from build123d import *

# Parameters (mm, degrees)
SKETCH1_W           = 5
SKETCH1_H           = 13
BOSS_EXTRUDE1_DEPTH = 2.5
SKETCH2_R           = 3
BOSS_EXTRUDE2_DEPTH = 5


with BuildPart() as part:
    # Sketch1 → Boss-Extrude1 (new body)
    with BuildSketch(Plane(origin=(0, 0, 0), x_dir=(1, 0, 0), z_dir=(0, 1, 0))):
        with Locations((2.5, 6.5)):
            Rectangle(SKETCH1_W, SKETCH1_H)
    extrude(amount=BOSS_EXTRUDE1_DEPTH)

    # Sketch2 → Boss-Extrude2 (add)
    with BuildSketch(Plane(origin=(0, 0, 0), x_dir=(1, 0, 0), z_dir=(0, 1, 0))):
        with Locations(Location((2.5, 10.335729582, 0), (0, 0, 270))):
            Circle(SKETCH2_R)
    extrude(amount=-BOSS_EXTRUDE2_DEPTH)


solid = part.part
For this review, take the finished solid that the model builds, in its own axes (mm). A direction names the side the tool comes from. Give positions to 0.01 mm unless a question says otherwise; leave off trailing zeros. Order: outer loops, then holes, each group sorted by start corner. A loop starts at its lowest first (then second) coordinate and runs counter-clockwise, first axis right, second up. Notation, with made-up numbers: (73.25, -17.75) -> (98.25, -17.75) arc R24 cw to (98.25, 4.25) -> close; hole circle Ø3 at (-11.75, 79.5). An arc over 180 degrees is marked (long way). Write item = value, one per line.
1) We need section A-A, the plane x = 4.85. Give the boundary of the cut face in (y, z), and give its area (3 significant figures).
Findings:
outline = (-5, -12.2) -> (0, -12.2) -> (0, -13) -> (2.5, -13) -> (2.5, 0) -> (0, 0) -> (0, -8.47) -> (-5, -8.47) -> close
area = 51.1 mm^2
2) To check wall thickness, follow L1, parallel to X at y = 1.5, z = -5.25; L2, parallel to Y at x = 2.75, z = -3.75; L3, parallel to Z at x = 4, y = 1.5. State the ranges of each line that lie inside material, in increasing order. Write a range as from..to.
Findings:
L1 = 0..5
L2 = 0..2.5
L3 = -13..0
3) We need section D-D, the plane z = -1.25. Give the boundary of the cut face in (x, y).
Findings:
outline = (0, 0) -> (5, 0) -> (5, 2.5) -> (0, 2.5) -> close
4) Insertion check: pin 1 (2 mm diameter, centred on x = 1, y = -2.5, fed in from +Z); pin 2 (1.2 mm diameter, centred on y = 1.5, z = -9.5, fed in from -X); pin 3 (1.2 mm diameter, centred on y = 1, z = -7, fed in from +X); pin 4 (1 mm diameter, centred on x = 4, y = 0.5, fed in from +Z). Each pin has a flat end and moves straight along its axis. Give the tip position at first contact, or say it passes through.
Findings:
pin_1 = -7.38
pin_2 = 0
pin_3 = 5
pin_4 = 0
5) We need section C-C, the plane y = -3. Give the boundary of the cut face in (x, z), and give its area (3 significant figures).
Findings:
outline = circle Ø6 at (2.5, -10.34)
area = 28.3 mm^2
6) We need section B-B, the plane z = -9.75. Give the boundary of the cut face in (x, y), and give its area (3 significant figures).
Findings:
outline = (-0.44, -5) -> (5.44, -5) -> (5.44, 0) -> (5, 0) -> (5, 2.5) -> (0, 2.5) -> (0, 0) -> (-0.44, 0) -> close
area = 41.9 mm^2
7) For faces 1 (the face through (0.3, 0, -12.7)), 2 (the face through (0, 1, -6)), 3 (the face through (2, 1, -13)), 4 (the face through (5, 1, -6)), 5 (the face through (4.528, -2.465, -12.547)), list the 3-axis set-ups (+Z, -Z, +X, -X, +Y, -Y) from which the entire face can be reached by the end or side of a thin tool; tool diameter is ignored.
Findings:
face_1 = -Z, -X, -Y
face_2 = +Z, -Z, -X, +Y
face_3 = -Z, +X, -X, +Y
face_4 = +Z, -Z, +X, +Y
face_5 = -Y
